For this review, take the finished solid that the model builds, in its own axes (mm). A direction names the side the tool comes from. Give positions to 0.01 mm unless a question says otherwise; leave off trailing zeros. Write each loop counter-clockwise with the first axis right and the second up, starting at its lowest first coordinate (ties: lowest second). Pieces come first, ordered by that corner, then holes.
Q1. Machinability: for faces 1 (the cylindrical face through (6.19, 30.42, 4.84)), 2 (the flat face through (27.029, 41.497, 5.07)), which of the approach directions +Z, -Z, +X, -X, +Y, -Y give a long, thin tool a straight path to every point of the face, cutting with its end or side? Answer none if there is none.
Q2. We need section B-B (y = 23). Write out the cut boundary in (x, z).
Q3. For line 1 (X direction, y = 31, z = 5); line 2 (X direction, y = 19, z = 5); line 3 (X direction, y = 42, z = 1), list the stretches that pass through material, from the lowest coordinate up.
Q4. Mouldability with a two-part tool opening along X and no side actions: class faces 3 (the flat face through (45.63, 16.63, 14.62)), 4 (the flat face through (0, 30, 7)), 5 (the cylindrical face through (11.07, 8.18, 5.07)) as released by +X, released by -X, zero draft, split by the parting line, or undercut.
Q5. We need section C-C (z = 5). Give the number of separate pieces and of enclosed holes in the cut face, then the cut area to 3 significant figures.
Q6. We need section D-D (x = 32). Write out the cut boundary in (y, z).
Q7. Insertion check: P1, Ø4, axis at x = 55, y = 12.5, coming from the -Z side; P2, Ø6, axis at x = 47.5, z = 15.5, coming from the +Y side; P3, Ø5, axis at x = 32.5, z = 18.5, coming from the +Y side. Each pin has a flat end and moves straight along its axis. Give the tip position at first contact, or say it passes through.
Q8. We need section A-A (z = 9). Write out the cut boundary in (x, y).
```python
from build123d import *

# Parameters (mm, degrees)
SKIZZE1_W                       = 90
SKIZZE1_H                       = 60
AUFSATZ_LINEAR_AUSTRAGEN1_DEPTH = 10
SCHNITT_LINEAR_AUSTRAGEN1_DEPTH = 10
SKIZZE3_R                       = 1.2
SCHNITT_LINEAR_AUSTRAGEN2_DEPTH = 68
AUFSATZ_LINEAR_AUSTRAGEN2_DEPTH = 90
SCHNITT_LINEAR_AUSTRAGEN4_DEPTH = 90


with BuildPart() as part:
    # Skizze1 → Aufsatz-Linear austragen1 (new body)
    with BuildSketch(Plane.XY):
        with Locations((45, 30)):
            Rectangle(SKIZZE1_W, SKIZZE1_H)
    extrude(amount=AUFSATZ_LINEAR_AUSTRAGEN1_DEPTH)

    # Skizze2 → Schnitt-Linear austragen1 (cut)
    with BuildSketch(Plane.XY.offset(10)):
        with BuildLine():
            Line((10, 50.05034464), (10, 9.94965536))
            ThreePointArc((10, 9.94965536), (11.096486968, 8.165372815), (13.183664201, 8.337532828))
            Line((13.183664201, 8.337532828), (40.491757454, 28.387877468))
            ThreePointArc((40.491757454, 28.387877468), (41.308093253, 30), (40.491757454, 31.612122532))
            Line((40.491757454, 31.612122532), (13.183664201, 51.662467172))
            ThreePointArc((13.183664201, 51.662467172), (11.096486968, 51.834627185), (10, 50.05034464))
        make_face()
        with BuildLine():
            Line((43.816335799, 35.160742066), (23.07733899, 50.387877468))
            ThreePointArc((23.07733899, 50.387877468), (22.360444711, 52.622798095), (24.261003191, 54))
            Line((24.261003191, 54), (65.738996809, 54))
            ThreePointArc((65.738996809, 54), (67.639555289, 52.622798095), (66.92266101, 50.387877468))
            Line((66.92266101, 50.387877468), (46.183664201, 35.160742066))
            ThreePointArc((46.183664201, 35.160742066), (45, 34.772864599), (43.816335799, 35.160742066))
        make_face()
        with BuildLine():
            Line((24.261003191, 6), (65.738996809, 6))
            ThreePointArc((65.738996809, 6), (67.639555289, 7.377201905), (66.92266101, 9.612122532))
            Line((66.92266101, 9.612122532), (46.183664201, 24.839257934))
            ThreePointArc((46.183664201, 24.839257934), (45, 25.227135401), (43.816335799, 24.839257934))
            Line((43.816335799, 24.839257934), (23.07733899, 9.612122532))
            ThreePointArc((23.07733899, 9.612122532), (22.360444711, 7.377201905), (24.261003191, 6))
        make_face()
        with BuildLine():
            Line((80, 50.05034464), (80, 9.94965536))
            ThreePointArc((80, 9.94965536), (78.903513032, 8.165372815), (76.816335799, 8.337532828))
            Line((76.816335799, 8.337532828), (49.508242546, 28.387877468))
            ThreePointArc((49.508242546, 28.387877468), (48.691906747, 30), (49.508242546, 31.612122532))
            Line((49.508242546, 31.612122532), (76.816335799, 51.662467172))
            ThreePointArc((76.816335799, 51.662467172), (78.903513032, 51.834627185), (80, 50.05034464))
        make_face()
    extrude(amount=-SCHNITT_LINEAR_AUSTRAGEN1_DEPTH, mode=Mode.SUBTRACT)

    # Skizze3 → Schnitt-Linear austragen2 (cut)
    with BuildSketch(Plane(origin=(0, 60, 0), x_dir=(1, 0, 0), z_dir=(0, 1, 0))):
        with Locations(Location((5, -5, 0), (0, 0, 270))):
            Circle(SKIZZE3_R)
        with Locations(Location((85, -5, 0), (0, 0, 270))):
            Circle(SKIZZE3_R)
    extrude(amount=-SCHNITT_LINEAR_AUSTRAGEN2_DEPTH, mode=Mode.SUBTRACT)

    # Skizze4 → Aufsatz-Linear austragen2 (add)
    with BuildSketch(Plane(origin=(90, 0, 0), x_dir=(0, 0, -1), z_dir=(1, 0, 0))):
        Polygon((-10, 60), (-10, 0), (-22.096946665, 43.542338596), align=None)
    extrude(amount=-AUFSATZ_LINEAR_AUSTRAGEN2_DEPTH)

    # Skizze5 → Schnitt-Linear austragen4 (cut)
    with BuildSketch(Plane(origin=(0, 60, 0), x_dir=(1, 0, 0), z_dir=(0, 1, 0))):
        Polygon((90, -14.917881766), (45, -22.096946665), (90, -22.096946665), align=None)
        Polygon((45, -22.096946665), (0, -14.917881766), (0, -22.096946665), align=None)
    extrude(amount=-SCHNITT_LINEAR_AUSTRAGEN4_DEPTH, mode=Mode.SUBTRACT)


solid = part.part
```
Computed:
1. face 1: +Y, -Y
1. face 2: -Z
2. outline: (0, 0) - (10, 0) - (10, 10) - (33.15, 10) - (33.15, 0) - (41.31, 0) - (41.31, 10) - (48.69, 10) - (48.69, 0) - (56.85, 0) - (56.85, 10) - (80, 10) - (80, 0) - (90, 0) - (90, 14.92) - (80.77, 16.39) - (9.23, 16.39) - (0, 14.92) - close; hole circle Ø2.4 at (5, 5); hole circle Ø2.4 at (85, 5)
3. line 1: x = 0 to 3.8, 6.2 to 10, 41.04 to 48.96, 80 to 83.8, 86.2 to 90
3. line 2: x = 0 to 3.8, 6.2 to 10, 27.71 to 35.86, 54.14 to 62.29, 80 to 83.8, 86.2 to 90
3. line 3: x = 0 to 10, 26.34 to 34.5, 55.5 to 63.66, 80 to 90
4. face 3: zero draft
4. face 4: released by -X
4. face 5: undercut
5. separate pieces: 3
5. enclosed holes: 4
5. area: 2,530 mm2
6. outline: (0, 0) - (6, 0) - (6, 10) - (16.16, 10) - (16.16, 0) - (22.15, 0) - (22.15, 10) - (37.85, 10) - (37.85, 0) - (43.84, 0) - (43.84, 10) - (54, 10) - (54, 0) - (60, 0) - (60, 10) - (46.36, 20.02) - (36.08, 20.02) - (0, 10) - close
7. P1: stops at z = 10
7. P2: stops at y = 56.6
7. P3: stops at y = 51.84
8. outline: (0, 0) - (90, 0) - (90, 60) - (0, 60) - close; hole (10, 9.95) arc R2 ccw to (13.18, 8.34) - (40.49, 28.39) arc R2 ccw to (40.49, 31.61) - (13.18, 51.66) arc R2 ccw to (10, 50.05) - close; hole (23.08, 9.61) arc R2 ccw to (24.26, 6) - (65.74, 6) arc R2 ccw to (66.92, 9.61) - (46.18, 24.84) arc R2 ccw to (43.82, 24.84) - close; hole (23.08, 50.39) - (43.82, 35.16) arc R2 ccw to (46.18, 35.16) - (66.92, 50.39) arc R2 ccw to (65.74, 54) - (24.26, 54) arc R2 ccw to start; hole (49.51, 28.39) - (76.82, 8.34) arc R2 ccw to (80, 9.95) - (80, 50.05) arc R2 ccw to (76.82, 51.66) - (49.51, 31.61) arc R2 ccw to start
